Job drawing, mm, ordinate dimensions from the low corner. One solid piece. Give positions to 0.01 mm unless a question says otherwise; leave off trailing zeros. Order: outer loops, then holes, each group sorted by start corner. A loop starts at its lowest first (then second) coordinate and runs counter-clockwise, first axis right, second up.
Item 1: Two-plate mould, pull along Z, no slides. Class the marked faces 1, 2, 3 and 4: released by +Z, released by -Z, zero draft, split by the parting line, or undercut.
Item 2: Band-saw the part on B-B on z = 7.5. Give the cut face in (x, y), plus the area to 3 significant figures.
Item 3: Band-saw the part on C-C on x = 7.5. Give the cut face in (y, z), plus the area to 3 significant figures.
Item 4: Band-saw the part on A-A on y = 9. Give the cut face in (x, z).
Item 5: Wall check: L1, parallel to Y at x = 3.25, z = 7.5; L2, parallel to Y at x = 8.75, z = 8.5; L3, parallel to Z at x = 6, y = 12.5. Give the ranges that are in metal, low to high.
Item 6: Flat gauge pin, fed straight in: P1, Ø3, axis at y = 11.5, z = 8, coming from the -X side. Where does the tip first touch, or does it go through?
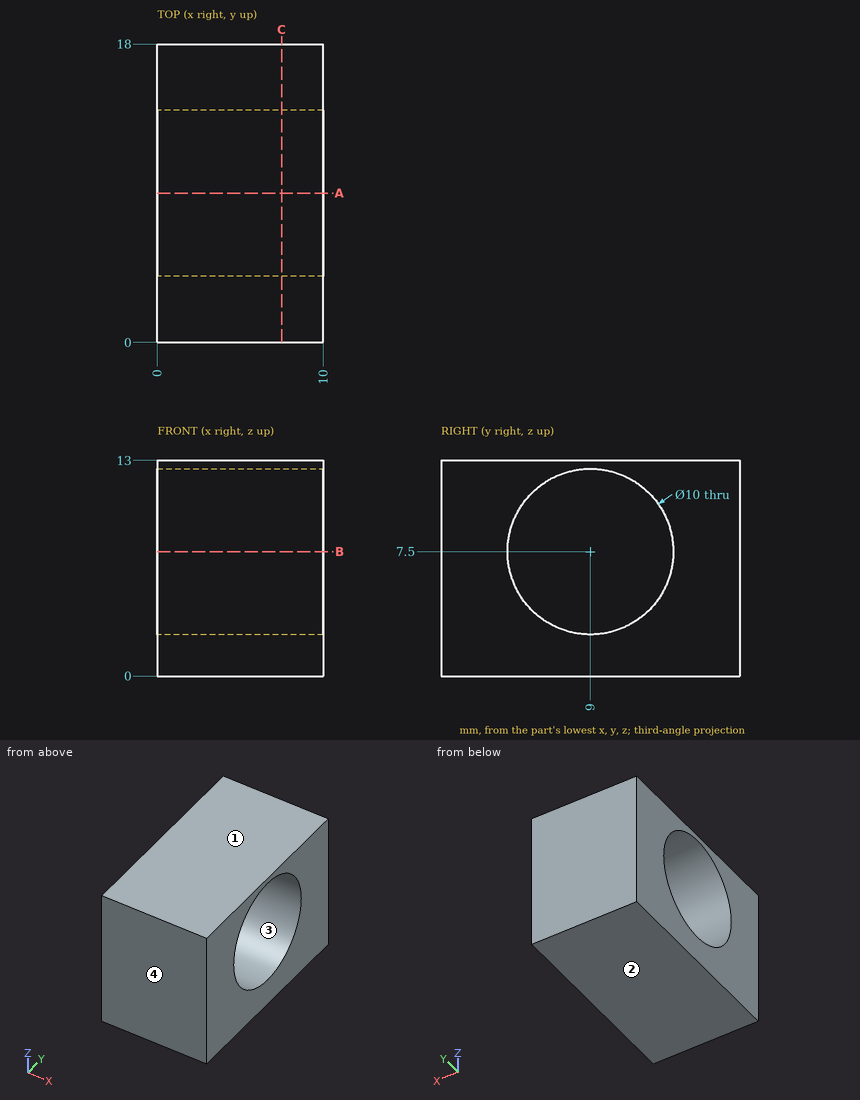
The answers:
1. face 1: released by +Z
1. face 2: released by -Z
1. face 3: undercut
1. face 4: zero draft
2. outline: (0, 0) - (10, 0) - (10, 4) - (0, 4) - close; (0, 14) - (10, 14) - (10, 18) - (0, 18) - close
2. area: 80.0 mm2
3. outline: (0, 0) - (18, 0) - (18, 13) - (0, 13) - close; hole circle Ø10 at (9, 7.5)
3. area: 155 mm2
4. outline: (0, 0) - (10, 0) - (10, 2.5) - (0, 2.5) - close; (0, 12.5) - (10, 12.5) - (10, 13) - (0, 13) - close
5. L1: y = 0 to 4, 14 to 18
5. L2: y = 0 to 4.1, 13.9 to 18
5. L3: z = 0 to 3.93, 11.07 to 13
6. P1: passes through
